Check sheet for the modelled part. Datum: model origin and axes. Units: mm. A direction names the side the tool comes from. Round coordinates to 2 decimals unless told otherwise and drop trailing zeros. Order: outer loops, then holes, each group sorted by start corner. A loop starts at its lowest first (then second) coordinate and runs counter-clockwise, first axis right, second up. Notation, with made-up numbers: M 79,49.5 L 90,49.5 A31 cw 90,81.5 Z; hole C -7,-12 d5. An arc over 180 degrees is marked long. One line per item, written item: value. Start each with the question number.
(1) Thickness scan on L1, parallel to Y at x = -41, z = 1; L2, parallel to X at y = 15.5, z = -17; L3, parallel to Y at x = 13, z = 4.5. Record the ranges inside material, lowest first.
(2) Release check for a two-part mould opening along Y. For faces 3 (the face through (41, 41, 30)), 4 (the face through (-1, -46.5, 2)), 5 (the face through (-1, 49.25, 2)) record: released by +Y, released by -Y, zero draft, split by the parting line, or undercut.
(3) Cross-section at A-A, the plane z = 25. Enter the section's corners in (x, y), and give its area (3 significant figures).
(4) Depth check by flat-ended pin: pin 1 Ø1 at (y, z) = (-26.5, -24) entering from +X; pin 2 Ø6 at (y, z) = (5, -47.5) entering from +X; pin 3 Ø10 at (x, z) = (24, -45.5) entering from -Y. Enter the tip coordinate at first touch or a pass-through.
(5) Access from +Z, -Z, +X, -X, +Y, -Y to the whole of each face (thin tool, end or side, straight path). Record for faces 1 (the face through (-24, 45, 0)), 2 (the face through (41, -41, 30)).
from build123d import *

# Parameters (mm, degrees)
SKIZZE1_W                       = 98.5
SKIZZE1_H                       = 98.5
SKIZZE1_W_2                     = 90.5
SKIZZE1_H_2                     = 90.5
AUFSATZ_LINEAR_AUSTRAGEN2_DEPTH = 5
SKIZZE6_W                       = 98.5
SKIZZE6_H                       = 98.5
AUFSATZ_LINEAR_AUSTRAGEN4_DEPTH = 60
AUFSATZ_LINEAR_AUSTRAGEN4_TAPER = 22
SKIZZE7_W                       = 93
SKIZZE7_H                       = 93
SCHNITT_LINEAR_AUSTRAGEN1_DEPTH = 5
SKIZZE10_R                      = 2
AUFSATZ_LINEAR_AUSTRAGEN5_DEPTH = 30


with BuildPart() as part:
    # Skizze1 → Aufsatz-Linear austragen2 (new body)
    # profile 1 of 5: a face of its own
    with BuildSketch(Plane.XY):
        Rectangle(SKIZZE1_W, SKIZZE1_H)
        Rectangle(SKIZZE1_W_2, SKIZZE1_H_2, mode=Mode.SUBTRACT)
    # profile 2 of 5: a face of its own
    with BuildSketch(Plane.XY):
        with BuildLine():
            Line((-45.25, 45.25), (-45.25, 21.270578271))
            ThreePointArc((-45.25, 21.270578271), (-35.355339059, 35.355339059), (-21.270578271, 45.25))
            Line((-21.270578271, 45.25), (-45.25, 45.25))
        make_face()
    # profile 3 of 5: a face of its own
    with BuildSketch(Plane.XY):
        with BuildLine():
            ThreePointArc((21.270578271, 45.25), (35.355339059, 35.355339059), (45.25, 21.270578271))
            Line((45.25, 21.270578271), (45.25, 45.25))
            Line((45.25, 45.25), (21.270578271, 45.25))
        make_face()
    # profile 4 of 5: a face of its own
    with BuildSketch(Plane.XY):
        with BuildLine():
            ThreePointArc((45.25, -21.270578271), (35.355339059, -35.355339059), (21.270578271, -45.25))
            Line((21.270578271, -45.25), (45.25, -45.25))
            Line((45.25, -45.25), (45.25, -21.270578271))
        make_face()
    # profile 5 of 5: a face of its own
    with BuildSketch(Plane.XY):
        with BuildLine():
            Line((-45.25, -21.270578271), (-45.25, -45.25))
            Line((-45.25, -45.25), (-21.270578271, -45.25))
            ThreePointArc((-21.270578271, -45.25), (-35.355339059, -35.355339059), (-45.25, -21.270578271))
        make_face()
    extrude(amount=AUFSATZ_LINEAR_AUSTRAGEN2_DEPTH)

    # Skizze6 → Aufsatz-Linear austragen4 (add)
    with BuildSketch(Plane(origin=(0, 0, 0), x_dir=(-1, 0, 0), z_dir=(0, 0, -1))):
        Rectangle(SKIZZE6_W, SKIZZE6_H)
    extrude(amount=AUFSATZ_LINEAR_AUSTRAGEN4_DEPTH, taper=AUFSATZ_LINEAR_AUSTRAGEN4_TAPER)

    # Schnitt-Ausformung4: read off the stored shape, not the designer's step
    # Schnitt-Ausformung4: loft between two sections, ruled curve by curve
    schnitt_ausformung4_from = [
        Edge.make_bspline([(45.25, 21.270578271, 0), (45.25, 17.725481893, 0), (45.25, 14.180385514, 0), (45.25, 7.090192757, 0), (45.25, 3.545096379, 0), (45.25, -3.545096379, 0), (45.25, -7.090192757, 0), (45.25, -14.180385514, 0), (45.25, -17.725481893, 0), (45.25, -21.270578271, 0)], [0, 0, 0, 0, 0.25, 0.25, 0.5, 0.5, 0.75, 0.75, 1, 1, 1, 1], 3),
        Edge.make_bspline([(21.270578271, -45.25, 0), (17.725481893, -45.25, 0), (14.180385514, -45.25, 0), (7.090192757, -45.25, 0), (3.545096379, -45.25, 0), (-3.545096379, -45.25, 0), (-7.090192757, -45.25, 0), (-14.180385514, -45.25, 0), (-17.725481893, -45.25, 0), (-21.270578271, -45.25, 0)], [0, 0, 0, 0, 0.25, 0.25, 0.5, 0.5, 0.75, 0.75, 1, 1, 1, 1], 3),
        Edge.make_bspline([(-45.25, -21.270578271, 0), (-45.25, -17.725481893, 0), (-45.25, -14.180385514, 0), (-45.25, -7.090192757, 0), (-45.25, -3.545096379, 0), (-45.25, 3.545096379, 0), (-45.25, 7.090192757, 0), (-45.25, 14.180385514, 0), (-45.25, 17.725481893, 0), (-45.25, 21.270578271, 0)], [0, 0, 0, 0, 0.25, 0.25, 0.5, 0.5, 0.75, 0.75, 1, 1, 1, 1], 3),
        Edge.make_bspline([(-21.270578271, 45.25, 0), (-17.725481893, 45.25, 0), (-14.180385514, 45.25, 0), (-7.090192757, 45.25, 0), (-3.545096379, 45.25, 0), (3.545096379, 45.25, 0), (7.090192757, 45.25, 0), (14.180385514, 45.25, 0), (17.725481893, 45.25, 0), (21.270578271, 45.25, 0)], [0, 0, 0, 0, 0.25, 0.25, 0.5, 0.5, 0.75, 0.75, 1, 1, 1, 1], 3),
        Edge.make_three_point_arc((21.270578271, -45.25, 0), (35.355339059, -35.355339059, 0), (45.25, -21.270578271, 0)),
        Edge.make_three_point_arc((-45.25, -21.270578271, 0), (-35.355339059, -35.355339059, 0), (-21.270578271, -45.25, 0)),
        Edge.make_three_point_arc((-21.270578271, 45.25, 0), (-35.355339059, 35.355339059, 0), (-45.25, 21.270578271, 0)),
        Edge.make_three_point_arc((45.25, 21.270578271, 0), (35.355339059, 35.355339059, 0), (21.270578271, 45.25, 0)),
    ]
    schnitt_ausformung4_to = [
        Edge.make_bspline([(18.5525, 8.720937091, -60), (19.17083125, 7.40552908, -60), (19.662710025, 5.991613705, -60), (20.327568653, 3.051483732, -60), (20.5, 1.525973244, -60), (20.5, -1.525973244, -60), (20.327568653, -3.051483732, -60), (19.662710025, -5.991613705, -60), (19.17083125, -7.40552908, -60), (18.5525, -8.720937091, -60)], [0, 0, 0, 0, 0.25, 0.25, 0.5, 0.5, 0.75, 0.75, 1, 1, 1, 1], 3),
        Edge.make_bspline([(8.720937091, -18.5525, -60), (7.40552908, -19.17083125, -60), (5.991613705, -19.662710025, -60), (3.051483732, -20.327568653, -60), (1.525973244, -20.5, -60), (-1.525973244, -20.5, -60), (-3.051483732, -20.327568653, -60), (-5.991613705, -19.662710025, -60), (-7.40552908, -19.17083125, -60), (-8.720937091, -18.5525, -60)], [0, 0, 0, 0, 0.25, 0.25, 0.5, 0.5, 0.75, 0.75, 1, 1, 1, 1], 3),
        Edge.make_bspline([(-18.5525, -8.720937091, -60), (-19.17083125, -7.40552908, -60), (-19.662710025, -5.991613705, -60), (-20.327568653, -3.051483732, -60), (-20.5, -1.525973244, -60), (-20.5, 1.525973244, -60), (-20.327568653, 3.051483732, -60), (-19.662710025, 5.991613705, -60), (-19.17083125, 7.40552908, -60), (-18.5525, 8.720937091, -60)], [0, 0, 0, 0, 0.25, 0.25, 0.5, 0.5, 0.75, 0.75, 1, 1, 1, 1], 3),
        Edge.make_bspline([(-8.720937091, 18.5525, -60), (-7.40552908, 19.17083125, -60), (-5.991613705, 19.662710025, -60), (-3.051483732, 20.327568653, -60), (-1.525973244, 20.5, -60), (1.525973244, 20.5, -60), (3.051483732, 20.327568653, -60), (5.991613705, 19.662710025, -60), (7.40552908, 19.17083125, -60), (8.720937091, 18.5525, -60)], [0, 0, 0, 0, 0.25, 0.25, 0.5, 0.5, 0.75, 0.75, 1, 1, 1, 1], 3),
        Edge.make_three_point_arc((8.720937091, -18.5525, -60), (14.495689014, -14.495689014, -60), (18.5525, -8.720937091, -60)),
        Edge.make_three_point_arc((-18.5525, -8.720937091, -60), (-14.495689014, -14.495689014, -60), (-8.720937091, -18.5525, -60)),
        Edge.make_three_point_arc((-8.720937091, 18.5525, -60), (-14.495689014, 14.495689014, -60), (-18.5525, 8.720937091, -60)),
        Edge.make_three_point_arc((18.5525, 8.720937091, -60), (14.495689014, 14.495689014, -60), (8.720937091, 18.5525, -60)),
    ]
    schnitt_ausformung4 = Solid(Shell([*[Face.make_surface_from_curves(schnitt_ausformung4_from[k], schnitt_ausformung4_to[k]) for k in range(8)], Face(Wire(schnitt_ausformung4_from)), Face(Wire(schnitt_ausformung4_to))]))
    add(schnitt_ausformung4, mode=Mode.SUBTRACT)

    # Skizze7 → Schnitt-Linear austragen1 (cut)
    with BuildSketch(Plane.XY):
        Rectangle(SKIZZE7_W, SKIZZE7_H)
    extrude(amount=SCHNITT_LINEAR_AUSTRAGEN1_DEPTH, mode=Mode.SUBTRACT)

    # Skizze10 → Aufsatz-Linear austragen5 (add)
    with BuildSketch(Plane.XY):
        with Locations((41.25, 41.25)):
            Circle(SKIZZE10_R)
        with Locations((41.25, -41.25)):
            Circle(SKIZZE10_R)
        with Locations((-41.25, -41.25)):
            Circle(SKIZZE10_R)
        with Locations((-41.25, 41.25)):
            Circle(SKIZZE10_R)
    extrude(amount=AUFSATZ_LINEAR_AUSTRAGEN5_DEPTH)


solid = part.part
Values found:
1. L1: -49.25 to -46.5, -43.23 to -39.27, 39.27 to 43.23, 46.5 to 49.25
1. L2: -42.38 to -37.81, 37.81 to 42.38
1. L3: -49.25 to -46.5, 46.5 to 49.25
2. face 3: zero draft
2. face 4: undercut
2. face 5: released by +Y
3. outline: C -41.25,-41.25 d4; C -41.25,41.25 d4; C 41.25,-41.25 d4; C 41.25,41.25 d4
3. area: 50.3 mm^2
4. pin 1: x = 39.76
4. pin 2: x = 31.27
4. pin 3: y = -32.89
5. face 1: +Z
5. face 2: +Z, +X, -X, +Y, -Y
